```python
from build123d import *

# Parameters (mm, degrees)
BOSS_EXTRU_1_DEPTH      = 5
ESQUISSE2_W             = 5
ESQUISSE2_H             = 10
ESQUISSE2_H_2           = 5
ESQUISSE2_W_2           = 10
ENL_V_MAT_EXTRU_1_DEPTH = 5
ESQUISSE3_W             = 18
ESQUISSE3_H             = 5
BOSS_EXTRU_2_DEPTH      = 5


with BuildPart() as part:
    # Esquisse1 → Boss.-Extru.1 (new body)
    with BuildSketch(Plane.XY):
        Polygon((0, 73), (42, 73), (42, 0), (0, 0), (0, 11.5), (32, 11.5), (32, 51), (0, 51), align=None)
    extrude(amount=BOSS_EXTRU_1_DEPTH)

    # Esquisse2 → Enlèv. mat.-Extru.1 (cut)
    with BuildSketch(Plane.XY.offset(5)):
        with Locations((2.5, 62)):
            Rectangle(ESQUISSE2_W, ESQUISSE2_H)
        with Locations((2.5, 5.75)):
            Rectangle(ESQUISSE2_W, ESQUISSE2_H_2)
        with Locations((34.5, 62)):
            Rectangle(ESQUISSE2_W, ESQUISSE2_H)
        with Locations((34.5, 5.75)):
            Rectangle(ESQUISSE2_W, ESQUISSE2_H_2)
        with Locations((19, 70.5)):
            Rectangle(ESQUISSE2_W_2, ESQUISSE2_H_2)
    extrude(amount=-ENL_V_MAT_EXTRU_1_DEPTH, mode=Mode.SUBTRACT)

    # Esquisse3 → Boss.-Extru.2 (add)
    with BuildSketch(Plane.XY.offset(5)):
        with Locations((19, 75.5)):
            Rectangle(ESQUISSE3_W, ESQUISSE3_H)
        with Locations((19, -2.5)):
            Rectangle(ESQUISSE3_W, ESQUISSE3_H)
    extrude(amount=-BOSS_EXTRU_2_DEPTH)


solid = part.part
```
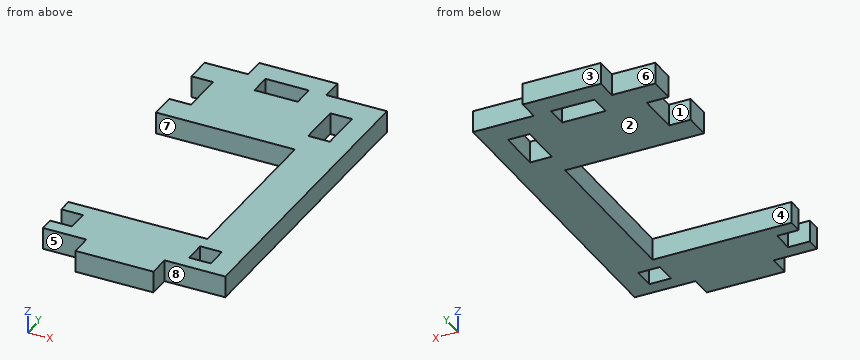
Geometry check sheet. Reference: the model listing, model coordinates, mm. Face numbers are marked on the shaded views. A direction names the side the tool comes from. Give positions to 0.01 mm unless a question says otherwise; leave off trailing zeros. Loops run counter-clockwise (first coordinate to the right, second up) from the corner with the lowest first, then second, coordinate; pieces in that order, holes last. Notation, with made-up numbers: M -39,-7 L 8,-7 A36 ccw 8,31 Z; hole C -35,36 d2. An arc over 180 degrees is marked long. Write item = value, one per line. Start each with the question number.
1. Section check D-D, the plane y = 27. Enter the section's corners in (x, z), plus the area to 3 significant figures.
2. Section check C-C, the plane z = 3.5. Give the number of separate pieces and of enclosed holes in the cut face, plus the area to 3 significant figures.
3. Section check A-A, the plane x = 11. Enter the section's corners in (y, z), plus the area to 4 significant figures.
4. Thickness scan on probe 1 along Y at (x, z) = (15, 4.7); probe 2 along Y at (x, z) = (36.5, 2.9); probe 3 along X at (y, z) = (71.5, 2.3). Record the ranges inside material, lowest first.
5. Tool access check on the marked faces 5, 6, 7 and 8. Record the directions out of +Z, -Z, +X, -X, +Y, -Y that give a thin tool (end or side, any length) a straight path to the whole face; none if there is none.
6. Draft check along Y on the marked faces 1, 2, 3 and 4. Enter one of: +Y half, -Y half, draft (parallel to the pull), parting line (faces both ways), or undercut.
7. Section check B-B, the plane x = 18. Enter the section's corners in (y, z).
8. Go/stop test with flat-tipped pins: P1, Ø2.5, axis at x = 36.5, z = 2, coming from the +Y side; P2, Ø1, axis at y = 59.5, z = 1.5, coming from the -X side. Record where each tip stops, or that it passes through.
Values follow:
q1.outline = M 32,0 L 42,0 L 42,5 L 32,5 Z
q1.area = 50.0 mm^2
q2.separate_pieces = 1
q2.enclosed_holes = 3
q2.area = 1,780 mm^2
q3.outline = M -5,0 L 11.5,0 L 11.5,5 L -5,5 Z; M 51,0 L 78,0 L 78,5 L 51,5 Z
q3.area = 217.5 mm^2
q4.probe_1 = -5 to 11.5, 51 to 68, 73 to 78
q4.probe_2 = 0 to 3.25, 8.25 to 57, 67 to 73
q4.probe_3 = 0 to 14, 24 to 42
q5.face_5 = +Z, -Z, -X, -Y
q5.face_6 = +Z, -Z, -X, +Y
q5.face_7 = +Z, -Z, -X
q5.face_8 = +Z, -Z, +X, -Y
q6.face_1 = undercut
q6.face_2 = draft
q6.face_3 = +Y half
q6.face_4 = undercut
q7.outline = M -5,0 L 11.5,0 L 11.5,5 L -5,5 Z; M 51,0 L 68,0 L 68,5 L 51,5 Z; M 73,0 L 78,0 L 78,5 L 73,5 Z
q8.P1 = 73
q8.P2 = 5
